For this review, take the finished solid that the model builds, in its own axes (mm). Face numbers are marked on the shaded views. A direction names the side the tool comes from. Coordinates: 2 decimals unless noted, no trailing zeros. Write each loop counter-clockwise with the first axis right and the second up, starting at its lowest first coordinate (ties: lowest second). Pieces come first, ordered by that corner, then holes. Notation, with made-up numbers: M 85,55 L 118,55 A31 ccw 118,92 Z; hole C 66,6.5 d3. An arc over 180 degrees is marked long. One line per question, with ' | ' between items.
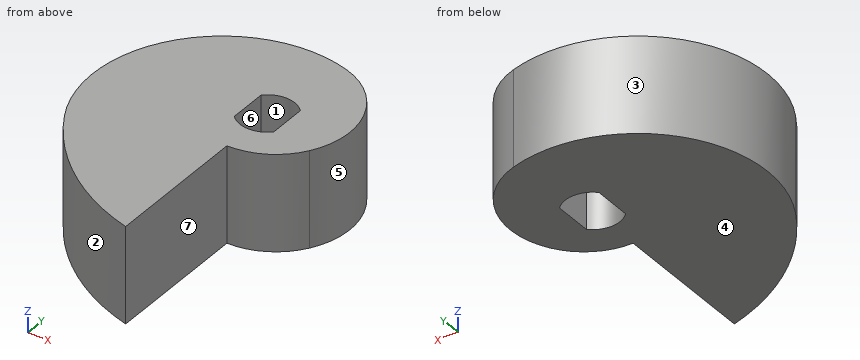
from build123d import *

# Parameters (mm, degrees)
EXTRUDE_448_DEPTH = 10


with BuildPart() as part:
    # Эскиз1 → Extrude 448 (new body)
    with BuildSketch(Plane.XY):
        with BuildLine():
            Line((0, -6), (0, -21))
            ThreePointArc((0, -21), (-8.058831333, -17.01600504), (-13.929161871, -10.207466455))
            ThreePointArc((-13.929161871, -10.207466455), (-12.703453351, 4.817077167), (1.681331293, 9.324542439))
            ThreePointArc((1.681331293, 9.324542439), (6.878554189, 4.4907399), (6.181719822, -2.572630025))
            ThreePointArc((6.181719822, -2.572630025), (3.534137975, -5.085826245), (0, -6))
        make_face()
        with BuildLine():
            Line((-2.05, 1.979898987), (-2.05, -1.979898987))
            ThreePointArc((-2.05, -1.979898987), (0, -2.85), (2.05, -1.979898987))
            Line((2.05, -1.979898987), (2.05, 1.979898987))
            ThreePointArc((2.05, 1.979898987), (0, 2.85), (-2.05, 1.979898987))
        make_face(mode=Mode.SUBTRACT)
    extrude(amount=EXTRUDE_448_DEPTH)


solid = part.part
1. Machinability: for the marked faces 5, 6 and 7, which of the approach directions +Z, -Z, +X, -X, +Y, -Y give a long, thin tool a straight path to every point of the face, cutting with its end or side? Answer none if there is none.
Computed values:
face 5: +Z, -Z, +X | face 6: +Z, -Z | face 7: +Z, -Z, +X, -Y
2. Draft analysis for pull direction Y (two halves, no side actions). For the marked faces 1, 2, 3 and 4, state which applies: pulls with the +Y half, pulls with the -Y half, needs draft (parallel to the pull), parting line crosses it, or undercut.
Computed values:
face 1: undercut | face 2: pulls with the -Y half | face 3: parting line crosses it | face 4: needs draft
3. Take a section at D-D on y = 8.5. State the section outline as (x, z) points.
Computed values:
outline: M -8.12,0 L 3.54,0 L 3.54,10 L -8.12,10 Z
4. Take a section at C-C on x = 5.25. State the section outline as (y, z) points.
Computed values:
outline: M -3.77,0 L 7.11,0 L 7.11,10 L -3.77,10 Z
5. For line 1 along Y through (x, z) = (1, 1); line 2 along Y through (x, z) = (0.5, 3); line 3 along X through (y, z) = (0, 8), list the stretches that pass through material, from the lowest coordinate up.
Computed values:
line 1: y = -5.93 to -2.67, 2.67 to 9.51 | line 2: y = -5.98 to -2.81, 2.81 to 9.62 | line 3: x = -15.16 to -2.05, 2.05 to 7.22
6. Take a section at A-A on z = 2.75. State the section outline as (x, y) points.
Computed values:
outline: M -13.93,-10.21 A22.62 ccw 0,-21 L 0,-6 A7.29 ccw 6.18,-2.57 A7.99 ccw 1.68,9.32 A13.49 ccw Z; hole M -2.05,-1.98 A2.85 ccw 2.05,-1.98 L 2.05,1.98 A2.85 ccw -2.05,1.98 Z
7. Clearance check with flat-ended pins moving along their axes: P1, Ø8, axis at x = 1, y = 1.5, coming from the -Z side; P2, Ø3, axis at y = -16.5, z = 3, coming from the +X side; P3, Ø5, axis at x = -9, z = 2, coming from the +Y side; P4, Ø2, axis at x = -11.5, z = 4, coming from the +Y side. State where each tip first meets the part, or that it passes through.
Computed values:
P1: stops at z = 0 | P2: stops at x = 0 | P3: stops at y = 9.17 | P4: stops at y = 7
8. Take a section at B-B on y = 2.5. State the section outline as (x, z) points, plus the area to 3 significant figures.
Computed values:
outline: M -14.2,0 L -1.37,0 L -1.37,10 L -14.2,10 Z; M 1.37,0 L 7.35,0 L 7.35,10 L 1.37,10 Z | area: 188 mm2
